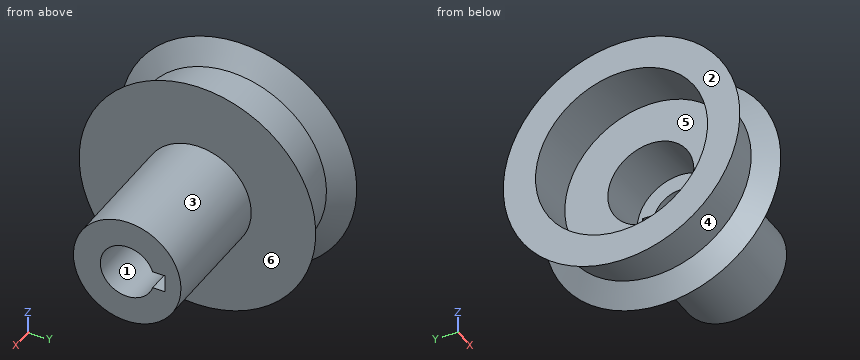
from build123d import *

# Parameters (mm, degrees)
CUT_EXTRUDE2_DEPTH = 123.780291578


with BuildPart() as part:
    # Sketch1 → Revolve1 (revolve)
    with BuildSketch(Plane(origin=(0, 0, 0), x_dir=(1, 0, 0), z_dir=(0, 1, 0)), mode=Mode.PRIVATE) as revolve1_sk:
        Polygon((95, 12.5), (95, 25), (35, 25), (35, 55), (28.060411696, 45), (7.5, 45), (0, 55), (0, 40), (25, 40), (25, 20), (50, 20), (50, 12.5), align=None)
    revolve(revolve1_sk.sketch.rotate(Axis((0, 0, 0), (1, 0, 0)), 180), axis=Axis((0, 0, 0), (1, 0, 0)))

    # Sketch3 → Cut-Extrude2 (cut, through all)
    with BuildSketch(Plane(origin=(95, 0, 0), x_dir=(0, 0, -1), z_dir=(1, 0, 0))):
        Polygon((0, 17.5), (-4, 17.5), (-4, 10.118492904), (4, 10.118492904), (4, 17.5), align=None)
    extrude(amount=-CUT_EXTRUDE2_DEPTH, mode=Mode.SUBTRACT)


solid = part.part
For this review, take the finished solid that the model builds, in its own axes (mm). Face numbers are marked on the shaded views. A direction names the side the tool comes from. Coordinates: 2 decimals unless noted, no trailing zeros. Write each loop counter-clockwise with the first axis right and the second up, starting at its lowest first coordinate (ties: lowest second). Pieces come first, ordered by that corner, then holes. Notation, with made-up numbers: (63, -23.5) -> (86, -23.5) arc R17 cw to (86, -17.5) -> close; hole circle Ø10 at (20, 85.5). An arc over 180 degrees is marked (long way). Write each question's results on one line, items separated by ' | '. Start each with the question number.
1) The part is to be moulded in two halves that separate along Y. For the marked faces 1, 2 and 3, say which applies: +Y half, -Y half, draft (parallel to the pull), parting line (faces both ways), or undercut.
2) Consider section B-B (z = 0). Write out the cut boundary in (x, y).
3) Consider section A-A (y = 0). Write out the cut boundary in (x, z), plus the area to 3 significant figures.
4) Consider section D-D (x = 21). Write out the cut boundary in (y, z), plus the area to 3 significant figures.
5) Consider section C-C (x = 56). Write out the cut boundary in (y, z), plus the area to 3 significant figures.
6) Insertion check: pin 1 (2 mm diameter, centred on y = 28.5, z = 28.5, fed in from +X); pin 2 (5 mm diameter, centred on x = 12, z = -11.5, fed in from +Y); pin 3 (3 mm diameter, centred on x = 26, z = -41.5, fed in from -Y); pin 4 (4 mm diameter, centred on y = 23.5, z = 42, fed in from -X). Each pin has a flat end and moves straight along its axis. Give the tip position at first contact, or say it passes through.
7) For the marked faces 4, 5 and 6, list the 3-axis set-ups (+Z, -Z, +X, -X, +Y, -Y) from which the entire face can be reached by the end or side of a thin tool; tool diameter is ignored.
8) Wall thickness on L1, parallel to Z at x = 83, y = 15; L2, parallel to Y at x = 60, z = 0; L3, parallel to Y at x = 18.75, z = 0: over which ranges is each line inside the solid? List them lowest first. Write a range as [from, to].
Geometry says:
1) face 1: undercut | face 2: draft | face 3: parting line
2) outline: (0, -55) -> (7.5, -45) -> (28.06, -45) -> (35, -55) -> (35, -25) -> (95, -25) -> (95, -12.5) -> (50, -12.5) -> (50, -20) -> (25, -20) -> (25, -40) -> (0, -40) -> close; (0, 40) -> (25, 40) -> (25, 20) -> (50, 20) -> (50, 17.5) -> (95, 17.5) -> (95, 25) -> (35, 25) -> (35, 55) -> (28.06, 45) -> (7.5, 45) -> (0, 55) -> close
3) outline: (0, -55) -> (7.5, -45) -> (28.06, -45) -> (35, -55) -> (35, -25) -> (95, -25) -> (95, -12.5) -> (50, -12.5) -> (50, -20) -> (25, -20) -> (25, -40) -> (0, -40) -> close; (0, 40) -> (25, 40) -> (25, 20) -> (50, 20) -> (50, 12.5) -> (95, 12.5) -> (95, 25) -> (35, 25) -> (35, 55) -> (28.06, 45) -> (7.5, 45) -> (0, 55) -> close | area: 2,170 mm^2
4) outline: circle Ø90 at (0, 0); hole circle Ø80 at (0, 0) | area: 1,340 mm^2
5) outline: circle Ø50 at (0, 0); hole (11.84, -4) -> (17.5, -4) -> (17.5, 4) -> (11.84, 4) arc R12.5 ccw (long way) to start | area: 1,430 mm^2
6) pin 1: x = 35 | pin 2: y = 44.09 | pin 3: y = -20.62 | pin 4: x = 0
7) face 4: none | face 5: -X | face 6: +X
8) L1: [-20, -4], [4, 20] | L2: [-25, -12.5], [17.5, 25] | L3: [-45, -40], [40, 45]
